Could you check a few things on this model? Use its own coordinates, in mm. A direction names the side the tool comes from. Give positions to 0.01 mm unless a question says otherwise; leave off trailing zeros. Loops run counter-clockwise (first coordinate to the right, second up) from the corner with the lowest first, then second, coordinate; pieces in that order, holes last.
1. Imagine slicing it at C-C (y = 10.75). List the corners of the cut face in (x, z) for me.
2. I need wall thicknesses on line 1 along Z through (x, y) = (-3, 6); line 2 along X through (y, z) = (2.75, -36); line 3 along X through (y, z) = (8, -8). Which ranges of each line are inside material? Lowest first, please.
3. Imagine slicing it at D-D (x = -27). List the corners of the cut face in (y, z) for me, plus the area to 3 significant figures.
4. Thinking about a two-plate mould opening in X: for faces 6 (the flat face through (-27, 10, -30)), 7 (the flat face through (0, 5, -20)), 8 (the cylindrical face through (-28.65, 3.7, -4.93)), which applies, +X half, -X half, draft (parallel to the pull), parting line (faces both ways), or undercut?
5. For P1, Ø5, axis at x = -27, z = -5, coming from the +Y side; P2, Ø1.3, axis at x = -26.5, y = 9, coming from the +Z side; P3, Ø2, axis at x = -27, z = -5, coming from the +Y side; P4, Ø3.5, axis at x = -27.5, y = 9.5, coming from the -Z side, each with a flat end and sliding along its axis, tell me the tip position at first contact or that it passes through.
6. For faces 1 (the flat face through (-30, 5, -20)), 2 (the flat face through (-28.4, 7.5, -6.2)), 3 (the flat face through (-25, 7.5, -35)), 4 (the flat face through (-1.6, 7.5, -6.2)), 5 (the flat face through (-4.4, 7.5, -36.2)), which set-ups out of +Z, -Z, +X, -X, +Y, -Y let a thin tool reach every point of the face, with its end or its side?
7. Imagine slicing it at B-B (y = 2.25). List the corners of the cut face in (x, z) for me.
8. Imagine slicing it at A-A (z = -35). List the corners of the cut face in (x, y) for me.
```python
from build123d import *

# Parameters (mm, degrees)
ESBO_O1_W                = 30
ESBO_O1_H                = 40
RESSALTO_EXTRUS_O1_DEPTH = 12
ESBO_O16_W               = 9.5
ESBO_O16_H               = 40
ESBO_O17_R               = 1.65
CORTE_EXTRUS_O12_DEPTH   = 13
CHANFRO1_SIZE            = 2
CHANFRO1_SIZE2           = 3.464101615
CHANFRO1_PART_2_SIZE     = 2
CHANFRO1_PART_2_SIZE2    = 3.464101615
CORTE_EXTRUS_O13_DEPTH   = 4.5


with BuildPart() as part:
    # Esboço1 → Ressalto-extrusão1 (new body)
    with BuildSketch(Plane(origin=(0, 0, 0), x_dir=(1, 0, 0), z_dir=(0, 1, 0))):
        with Locations((-15, 20)):
            Rectangle(ESBO_O1_W, ESBO_O1_H)
    extrude(amount=RESSALTO_EXTRUS_O1_DEPTH)

    # Esboço16 → Corte-Revolução1 (revolve, cut)
    with BuildSketch(Plane.XZ):
        with Locations((-19.75, -20)):
            Rectangle(ESBO_O16_W, ESBO_O16_H)
    revolve(axis=Axis((-15, 0, -40), (0, 0, 1)), mode=Mode.SUBTRACT)

    # Esboço17 → Corte-extrusão12 (cut, through all)
    with BuildSketch(Plane.XZ):
        with Locations((-27, -35)):
            Circle(ESBO_O17_R)
        with Locations((-27, -5)):
            Circle(ESBO_O17_R)
        with Locations((-3, -35)):
            Circle(ESBO_O17_R)
        with Locations((-3, -5)):
            Circle(ESBO_O17_R)
    extrude(amount=-CORTE_EXTRUS_O12_DEPTH, mode=Mode.SUBTRACT)

    # Chanfro1
    chanfro1_edges = [part.edges().sort_by_distance(p)[0] for p in [
        (0, 6, 0),
        (0, 6, -40),
    ]]
    chanfro1_side = [part.faces().sort_by_distance(p)[0] for p in [
        (0, 6, -20),
    ]]
    chamfer(chanfro1_edges, length=CHANFRO1_SIZE, length2=CHANFRO1_SIZE2, reference=chanfro1_side[0])

    # Chanfro1 part 2
    chanfro1_part_2_edges = [part.edges().sort_by_distance(p)[0] for p in [
        (-30, 6, 0),
        (-30, 6, -40),
    ]]
    chanfro1_part_2_side = [part.faces().sort_by_distance(p)[0] for p in [
        (-30, 6, -20),
    ]]
    chamfer(chanfro1_part_2_edges, length=CHANFRO1_PART_2_SIZE, length2=CHANFRO1_PART_2_SIZE2, reference=chanfro1_part_2_side[0])

    # Esboço18 → Corte-extrusão13 (cut)
    with BuildSketch(Plane(origin=(0, 12, 0), x_dir=(1, 0, 0), z_dir=(0, 1, 0))):
        Polygon((-6, 40), (-6, 30), (0, 30), (0, 38), (-3.464101615, 40), align=None)
        Polygon((-24, 40), (-26.535898385, 40), (-30, 38), (-30, 30), (-24, 30), align=None)
        Polygon((0, 10), (0, 2), (-3.464101615, 0), (-6, 0), (-6, 10), align=None)
        Polygon((-24, 0), (-24, 10), (-30, 10), (-30, 2), (-26.535898385, 0), align=None)
    extrude(amount=-CORTE_EXTRUS_O13_DEPTH, mode=Mode.SUBTRACT)


solid = part.part
```
Derived:
1. outline: (-30, -30) - (-24, -30) - (-24, -40) - (-6, -40) - (-6, -30) - (0, -30) - (0, -10) - (-6, -10) - (-6, 0) - (-24, 0) - (-24, -10) - (-30, -10) - close
2. line 1: z = -39.73 to -36.65, -33.35 to -6.65, -3.35 to -0.27
2. line 2: x = -30 to -28.31, -25.69 to -24.09, -5.91 to -4.31, -1.69 to 0
2. line 3: x = -24 to -20.12, -9.88 to -6
3. outline: (0, -39.73) - (7.5, -39.73) - (7.5, -36.65) - (0, -36.65) - close; (0, -33.35) - (7.5, -33.35) - (7.5, -30) - (12, -30) - (12, -10) - (7.5, -10) - (7.5, -6.65) - (0, -6.65) - close; (0, -3.35) - (7.5, -3.35) - (7.5, -0.27) - (0, -0.27) - close
3. area: 336 mm2
4. face 6: draft
4. face 7: +X half
4. face 8: undercut
5. P1: stops at y = 7.5
5. P2: stops at z = -10
5. P3: passes through
5. P4: stops at z = -30
6. face 1: +Z, -Z, -X, +Y, -Y
6. face 2: +Z, -X, +Y
6. face 3: -Z, -X, +Y
6. face 4: +Z, +X, +Y
6. face 5: -Z, +X, +Y
7. outline: (-30, -38) - (-26.54, -40) - (-24.23, -40) - (-24.23, 0) - (-26.54, 0) - (-30, -2) - close; (-5.77, -40) - (-3.46, -40) - (0, -38) - (0, -2) - (-3.46, 0) - (-5.77, 0) - close; hole circle Ø3.3 at (-27, -35); hole circle Ø3.3 at (-27, -5); hole circle Ø3.3 at (-3, -35); hole circle Ø3.3 at (-3, -5)
8. outline: (-30, 0) - (-28.65, 0) - (-28.65, 7.5) - (-30, 7.5) - close; (-25.35, 0) - (-24.5, 0) arc R9.5 cw to (-5.5, 0) - (-4.65, 0) - (-4.65, 7.5) - (-6, 7.5) - (-6, 12) - (-24, 12) - (-24, 7.5) - (-25.35, 7.5) - close; (-1.35, 0) - (0, 0) - (0, 7.5) - (-1.35, 7.5) - close
